Geometry check sheet. Reference: the model listing, model coordinates, mm. A direction names the side the tool comes from. Coordinates: 2 decimals unless noted, no trailing zeros. Order: outer loops, then holes, each group sorted by start corner. A loop starts at its lowest first (then second) coordinate and runs counter-clockwise, first axis right, second up. Notation, with made-up numbers: M -35.75,39.25 L 6.25,39.25 A13 cw 6.25,63.25 Z; hole C 77,63 d6. An arc over 180 degrees is marked long. One line per item, written item: value. Start each with the question number.
1) Sectioned sample at D-D, the plane x = -10.5. Enter the section's corners in (y, z), then the cut area to 3 significant figures.
2) Draft check along X on faces 1 (the flat face through (7, -1, -37)), 2 (the flat face through (-26.5, -1, 11)), 3 (the flat face through (7, -1, -39)). Enter one of: pulls with the +X half, pulls with the -X half, needs draft (parallel to the pull), parting line crosses it, or undercut.
3) Go/stop test with a flat-tipped pin: P1, Ø6, axis at x = 22, z = -6, coming from the -Y side. Record where the tip stops, or that it passes through.
4) Access from +Z, -Z, +X, -X, +Y, -Y to the whole of each face (thin tool, end or side, straight path). Record for faces 4 (the flat face through (22, 2, 23)), 5 (the flat face through (-24.5, -1, 11)).
5) Thickness scan on L1, parallel to X at y = 1.5, z = 11.25; L2, parallel to X at y = -1, z = 17.5; L3, parallel to Z at x = -5.5, y = -0.3. Record the ranges inside material, lowest first. Write a range as from..to.
6) Sectioned sample at A-A, the plane z = 11.25. Enter the section's corners in (x, y), then the cut area to 3 significant figures.
7) Sectioned sample at B-B, the plane x = 7.75. Enter the section's corners in (y, z), then the cut area to 3 significant figures.
8) Sectioned sample at C-C, the plane y = -1.95. Enter the section's corners in (x, z).
```python
from build123d import *

# Parameters (mm, degrees)
CROQUIS1_W                   = 64.5
CROQUIS1_H                   = 96.5
CROQUIS1_R                   = 16
SALIENTE_EXTRUIR4_DEPTH      = 2
CROQUIS2_W                   = 68.5
CROQUIS2_H                   = 100.5
CROQUIS2_W_2                 = 64.5
CROQUIS2_H_2                 = 96.5
SALIENTE_EXTRUIR5_DEPTH      = 3
SALIENTE_EXTRUIR5_DEPTH_BACK = 2


with BuildPart() as part:
    # Croquis1 → Saliente-Extruir4 (new body)
    with BuildSketch(Plane(origin=(0, 0, 0), x_dir=(1, 0, 0), z_dir=(0, 1, 0))):
        with Locations((7.75, -11.25)):
            Rectangle(CROQUIS1_W, CROQUIS1_H)
        with Locations((7.75, -11.25)):
            Circle(CROQUIS1_R, mode=Mode.SUBTRACT)
    extrude(amount=SALIENTE_EXTRUIR4_DEPTH)

    # Croquis2 → Saliente-Extruir5 (add, two sides)
    with BuildSketch(Plane.XZ) as saliente_extruir5_sk:
        with Locations((7.75, 11.25)):
            Rectangle(CROQUIS2_W, CROQUIS2_H)
        with Locations((7.75, 11.25)):
            Rectangle(CROQUIS2_W_2, CROQUIS2_H_2, mode=Mode.SUBTRACT)
    extrude(amount=SALIENTE_EXTRUIR5_DEPTH)
    extrude(saliente_extruir5_sk.sketch, amount=-SALIENTE_EXTRUIR5_DEPTH_BACK)


solid = part.part
```
Final values:
1. outline: M -3,-39 L 2,-39 L 2,61.5 L -3,61.5 L -3,59.5 L 0,59.5 L 0,-37 L -3,-37 Z
1. area: 213 mm^2
2. face 1: undercut
2. face 2: pulls with the -X half
2. face 3: needs draft
3. P1: stops at y = 0
4. face 4: +Z, -Z, +X, -X, +Y
4. face 5: -Y
5. L1: x = -26.5..-8.25, 23.75..42
5. L2: x = -26.5..-24.5, 40..42
5. L3: z = -39..-37, 59.5..61.5
6. outline: M -26.5,-3 L -24.5,-3 L -24.5,0 L -8.25,0 L -8.25,2 L -26.5,2 Z; M 23.75,0 L 40,0 L 40,-3 L 42,-3 L 42,2 L 23.75,2 Z
6. area: 85.0 mm^2
7. outline: M -3,-39 L 2,-39 L 2,-4.75 L 0,-4.75 L 0,-37 L -3,-37 Z; M -3,59.5 L 0,59.5 L 0,27.25 L 2,27.25 L 2,61.5 L -3,61.5 Z
7. area: 149 mm^2
8. outline: M -26.5,-39 L 42,-39 L 42,61.5 L -26.5,61.5 Z; hole M -24.5,-37 L 40,-37 L 40,59.5 L -24.5,59.5 Z
